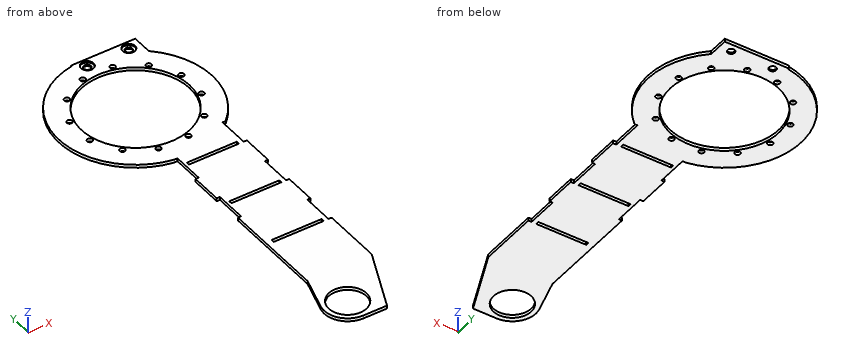
```python
from build123d import *

# Parameters (mm, degrees)
SKETCH_1_R                   = 12
SKETCH_1_W                   = 32
SKETCH_1_H                   = 2
SKETCH_1_R_2                 = 1.7
SKETCH_1_R_3                 = 34.5
EXTRUDE_1_DEPTH              = 2
HOLE_WIZARD_M4_1_D           = 4.5
HOLE_WIZARD_M4_1_CBORE_D     = 8
HOLE_WIZARD_M4_1_CBORE_DEPTH = 1


with BuildPart() as part:
    # 草图1 → 凸台-拉伸1 (new body)
    with BuildSketch(Plane.XY):
        with BuildLine():
            ThreePointArc((-8, 48.342527861), (-49, 0), (-8, -48.342527861))
            Line((-8, -48.342527861), (-6, -48.342527861))
            Line((-6, -48.342527861), (-6, -68.342527861))
            Line((-6, -68.342527861), (-8, -68.342527861))
            Line((-8, -68.342527861), (-8, -88.342527861))
            Line((-8, -88.342527861), (-6, -88.342527861))
            Line((-6, -88.342527861), (-6, -108.342527861))
            Line((-6, -108.342527861), (-8, -108.342527861))
            Line((-8, -108.342527861), (-8, -128.342527861))
            Line((-8, -128.342527861), (-8, -174))
            Line((-8, -174), (-14.392579, -195.774639692))
            ThreePointArc((-14.392579, -195.774639692), (-12.007922481, -208.989426995), (0, -215))
            Line((0, -215), (15, -215))
            Line((15, -215), (33, -174))
            Line((33, -174), (33, -136.221540553))
            Line((33, -136.221540553), (31, -136.221540553))
            Line((31, -136.221540553), (31, -116.221540553))
            Line((31, -116.221540553), (33, -116.221540553))
            Line((33, -116.221540553), (33, -96.221540553))
            Line((33, -96.221540553), (31, -96.221540553))
            Line((31, -96.221540553), (31, -76.221540553))
            Line((31, -76.221540553), (33, -76.221540553))
            Line((33, -76.221540553), (33, -56.221540553))
            Line((33, -56.221540553), (31, -56.221540553))
            Line((31, -56.221540553), (31, -36.221540553))
            Line((31, -36.221540553), (33, -36.221540553))
            ThreePointArc((33, -36.221540553), (49, 0), (33, 36.221540553))
            Line((33, 36.221540553), (33, 49))
            Line((33, 49), (-8, 49))
            Line((-8, 49), (-8, 48.342527861))
        make_face()
        with Locations((0, -200)):
            Circle(SKETCH_1_R, mode=Mode.SUBTRACT)
        with Locations((12, -135.221540553)):
            Rectangle(SKETCH_1_W, SKETCH_1_H, mode=Mode.SUBTRACT)
        with Locations((12, -95.221540553)):
            Rectangle(SKETCH_1_W, SKETCH_1_H, mode=Mode.SUBTRACT)
        with Locations((-26.162950904, -26.162950904)):
            Circle(SKETCH_1_R_2, mode=Mode.SUBTRACT)
        with Locations((-9.576304669, -35.739255573)):
            Circle(SKETCH_1_R_2, mode=Mode.SUBTRACT)
        with Locations((-35.739255573, -9.576304669)):
            Circle(SKETCH_1_R_2, mode=Mode.SUBTRACT)
        with Locations((-35.739255573, 9.576304669)):
            Circle(SKETCH_1_R_2, mode=Mode.SUBTRACT)
        with Locations((-26.162950904, 26.162950904)):
            Circle(SKETCH_1_R_2, mode=Mode.SUBTRACT)
        Circle(SKETCH_1_R_3, mode=Mode.SUBTRACT)
        with Locations((-9.576304669, 35.739255573)):
            Circle(SKETCH_1_R_2, mode=Mode.SUBTRACT)
        with Locations((12, -55.221540553)):
            Rectangle(SKETCH_1_W, SKETCH_1_H, mode=Mode.SUBTRACT)
        with Locations((9.576304669, -35.739255573)):
            Circle(SKETCH_1_R_2, mode=Mode.SUBTRACT)
        with Locations((26.162950904, -26.162950904)):
            Circle(SKETCH_1_R_2, mode=Mode.SUBTRACT)
        with Locations((9.576304669, 35.739255573)):
            Circle(SKETCH_1_R_2, mode=Mode.SUBTRACT)
        with Locations((35.739255573, -9.576304669)):
            Circle(SKETCH_1_R_2, mode=Mode.SUBTRACT)
        with Locations((35.739255573, 9.576304669)):
            Circle(SKETCH_1_R_2, mode=Mode.SUBTRACT)
        with Locations((26.162950904, 26.162950904)):
            Circle(SKETCH_1_R_2, mode=Mode.SUBTRACT)
    extrude(amount=EXTRUDE_1_DEPTH)

    # M4 六角凹头盖的柱孔1 (through all)
    with Locations(Plane(origin=(-1, 44, 2), x_dir=(1, 0, 0), z_dir=(0, 0, 1))):
        with Locations((0, 0), (26.5, 0)):
            CounterBoreHole(HOLE_WIZARD_M4_1_D / 2, HOLE_WIZARD_M4_1_CBORE_D / 2, HOLE_WIZARD_M4_1_CBORE_DEPTH)


solid = part.part
```
Design review of the part built by this model. Coordinates are the model's own, in mm. Give positions to 0.01 mm unless a question says otherwise; leave off trailing zeros. Order: outer loops, then holes, each group sorted by start corner. A loop starts at its lowest first (then second) coordinate and runs counter-clockwise, first axis right, second up. Notation, with made-up numbers: (66.25, 55.5) -> (113.25, 55.5) arc R20 ccw to (113.25, 79.5) -> close; hole circle Ø2 at (-38, 18.5). An arc over 180 degrees is marked (long way). Write item = value, one per line. Start each with the question number.
(1) For pin 1 (0.6 mm diameter, centred on y = 44.5, z = 0.5, fed in from +X); pin 2 (1 mm diameter, centred on y = -41.5, z = 1, fed in from -X); pin 3 (2.5 mm diameter, centred on x = -26.16, y = -26.16, fed in from -Z); pin 4 (0.6 mm diameter, centred on x = 32, z = 0.5, fed in from -Y), all flat-tipped, find the tip position at first contact; note any pin that passes through.
(2) We need section A-A on y = 0. Write out the cut boundary in (x, z).
(3) We need section D-D on z = 0.4. State how many separate pieces and enclosed holes the cut face has, plus the area to 3 significant figures.
(4) To check wall thickness, follow line 1 along Y through (x, z) = (4, 1.65); line 2 along X through (y, z) = (27, 0.95); line 3 along Y through (x, z) = (15, 0.45). State the ranges of each line that lie inside material, in increasing order.
(5) We need section B-B on y = -200. Write out the cut boundary in (x, z), plus the area to 3 significant figures.
(6) We need section C-C on y = -141.5. Write out the cut boundary in (x, z).
Numbers:
q1.pin_1 = 33
q1.pin_2 = -26.83
q1.pin_3 = through
q1.pin_4 = -176.96
q2.outline = (-49, 0) -> (-34.5, 0) -> (-34.5, 2) -> (-49, 2) -> close; (34.5, 0) -> (49, 0) -> (49, 2) -> (34.5, 2) -> close
q3.separate_pieces = 1
q3.enclosed_holes = 19
q3.area = 9,680 mm^2
q4.line_1 = -215 to -211.31, -188.69 to -136.22, -134.22 to -96.22, -94.22 to -56.22, -54.22 to -34.27, 34.27 to 49
q4.line_2 = -40.89 to -27.64, -24.68 to -21.48, 21.48 to 24.68, 27.64 to 40.89
q4.line_3 = -215 to -136.22, -134.22 to -96.22, -94.22 to -56.22, -54.22 to -31.07, 31.07 to 49
q5.outline = (-15, 0) -> (-12, 0) -> (-12, 2) -> (-15, 2) -> close; (12, 0) -> (21.59, 0) -> (21.59, 2) -> (12, 2) -> close
q5.area = 25.2 mm^2
q6.outline = (-8, 0) -> (33, 0) -> (33, 2) -> (-8, 2) -> close
